Can you work these out from the model? Positions are in its coordinate system, mm. Give positions to 0.01 mm unless a question says otherwise; leave off trailing zeros. Order: outer loops, then holes, each group sorted by start corner. A loop starts at its lowest first (then second) coordinate and runs counter-clockwise, first axis right, second up. Notation, with made-up numbers: M 72,78.5 L 83,78.5 A35 ccw 83,113.5 Z; hole C 73.25,-38.5 d10. An arc over 180 degrees is marked long. One line per question, with ' | ' between items. Start each with the question number.
1) If we section it at C-C, the plane z = 11: Please give me the cut outline in (x, y), plus the area to 3 significant figures.
2) If we section it at A-A, the plane x = 14: Please give me the cut outline in (y, z), plus the area to 3 significant figures.
3) If we section it at B-B, the plane y = 60: Please give me the cut outline in (x, z), plus the area to 3 significant figures.
4) If we section it at D-D, the plane x = 34.1: Please give me the cut outline in (y, z), plus the area to 3 significant figures.
5) I'm going to push flat-ended pins straight in: pin 1 Ø1.5 at (y, z) = (5.5, 22) entering from -X; pin 2 Ø6 at (x, z) = (9, 30) entering from -Y; pin 3 Ø8 at (y, z) = (4, 30.5) entering from +X. Where does each tip first touch, or does it pass through?
6) Please list where these lines run through material, in increasing order: line 1 along Y through (x, z) = (32.5, 46.5); line 2 along X through (y, z) = (72, 77.5); line 3 along X through (y, z) = (37.5, 15.5). Write a range as [from, to].
```python
from build123d import *

# Parameters (mm, degrees)
BOSS_EXTRUDE1_DEPTH = 78.5
SKETCH4_R           = 17.5
BOSS_EXTRUDE2_DEPTH = 12.5
BOSS_EXTRUDE2_TAPER = 8
FILLET1_R           = 1
FILLET2_R           = 1
CHAMFER1_SIZE       = 2
CHAMFER2_SIZE       = 8
CHAMFER2_SIZE_2     = 8.365483885


with BuildPart() as part:
    # Sketch1 → Boss-Extrude1 (new body)
    with BuildSketch(Plane(origin=(0, 0, 0), x_dir=(1, 0, 0), z_dir=(0, 1, 0))):
        Polygon((0, 0), (68.2, 0), (64, -98.1), (4.2, -98.1), align=None)
    extrude(amount=BOSS_EXTRUDE1_DEPTH)

    # Sketch4 → Boss-Extrude2 (add)
    with BuildSketch(Plane.XZ):
        with Locations((34.1, 73.6)):
            Circle(SKETCH4_R)
    extrude(amount=BOSS_EXTRUDE2_DEPTH, taper=BOSS_EXTRUDE2_TAPER)

    # Fillet1
    fillet1_edges = [part.edges().sort_by_distance(p)[0] for p in [
        (18.356760434, -12.5, 73.6),
    ]]
    fillet(fillet1_edges, radius=FILLET1_R)

    # Fillet2
    fillet2_edges = [part.edges().sort_by_distance(p)[0] for p in [
        (16.6, 0, 73.6),
    ]]
    fillet(fillet2_edges, radius=FILLET2_R)

    # Chamfer1
    chamfer1_edges = [part.edges().sort_by_distance(p)[0] for p in [
        (66.1, 0, 49.05),
        (34.1, 0, 98.1),
        (2.1, 0, 49.05),
    ]]
    chamfer(chamfer1_edges, length=CHAMFER1_SIZE)

    # Chamfer2
    # the kernel refuses this chamfer: 8.365483885, 8 mm, written as the material it takes off along each edge
    with BuildSketch(Plane(origin=(4.2, -19.537429792, 98.1), x_dir=(-0.07144532061930704, 0, -0.9974445178362575), z_dir=(0, 1, 0))) as chamfer2_piece_1:
        Polygon((CHAMFER2_SIZE * 0.999587640261, -CHAMFER2_SIZE * 0.028714968879), (-CHAMFER2_SIZE_2 * 0.071445320615, -CHAMFER2_SIZE_2 * 0.997444517777), (0, 0), align=None)
    extrude(amount=119.574859584, mode=Mode.SUBTRACT)
    with BuildSketch(Plane(origin=(64, -19.537429792, 98.1), x_dir=(0.06900069983757576, 0, -0.9976166114404496), z_dir=(0, 1, 0))) as chamfer2_piece_2:
        Polygon((CHAMFER2_SIZE_2 * 0.999655009427, CHAMFER2_SIZE_2 * 0.0262652243269), (-CHAMFER2_SIZE * 0.0690006998376, CHAMFER2_SIZE * 0.99761661144), (0, 0), align=None)
    extrude(amount=119.574859584, mode=Mode.SUBTRACT)


solid = part.part
```
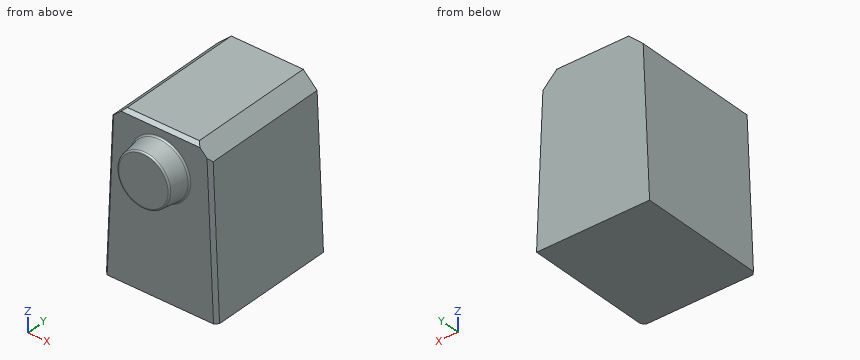
Results found:
1) outline: M 0.47,2 L 2.47,0 L 65.73,0 L 67.73,2 L 67.73,78.5 L 0.47,78.5 Z | area: 5,280 mm²
2) outline: M 0,0 L 78.5,0 L 78.5,98.1 L 2,98.1 L 0,96.1 Z | area: 7,700 mm²
3) outline: M 0,0 L 68.2,0 L 64.36,89.74 L 56,98.1 L 12.57,98.1 L 3.86,90.11 Z | area: 6,210 mm²
4) outline: M -12.5,58.73 A1 ccw -11.64,57.74 L -0.86,56.22 A1 cw 0,55.23 L 0,0 L 78.5,0 L 78.5,98.1 L 2,98.1 L 0,96.1 L 0,91.97 A1 cw -0.86,90.98 L -11.64,89.46 A1 ccw -12.5,88.47 Z | area: 8,110 mm²
5) pin 1: stops at x = 0.91 | pin 2: stops at y = 0 | pin 3: stops at x = 67.07
6) line 1: y = [0, 78.5] | line 2: x = [3.32, 64.88] | line 3: x = [0.66, 67.54]
